The drawing under review shows one solid part. Ordinate dimensions are in mm from its lowest x, y, z. Round coordinates to 2 decimals unless told otherwise and drop trailing zeros. Order: outer loops, then holes, each group sorted by start corner. A loop starts at its lowest first (then second) coordinate and runs counter-clockwise, first axis right, second up. Notation, with made-up numbers: M 81.5,55 L 107.5,55 A27 ccw 107.5,92 Z; hole C -25,-18 d10. An arc over 180 degrees is marked long. Answer as a JSON object with one key per item and string values. Group by question number.
1) Consider section A-A, the plane x = 20. Write out the cut boundary in (y, z).
2) Consider section B-B, the plane z = 0.35. Write out the cut boundary in (x, y).
3) To check wall thickness, follow line 1 (Y direction, x = 60, z = 0.65); line 2 (X direction, y = 24, z = 0.8); line 3 (Y direction, x = 23, z = 0.35). State the ranges of each line that lie inside material, in increasing order.
4) Insertion check: pin 1 Ø7 at (x, y) = (60, 60) entering from -Z. The pin has a flat end and moves straight along its axis. Give the tip position at first contact, or say it passes through.
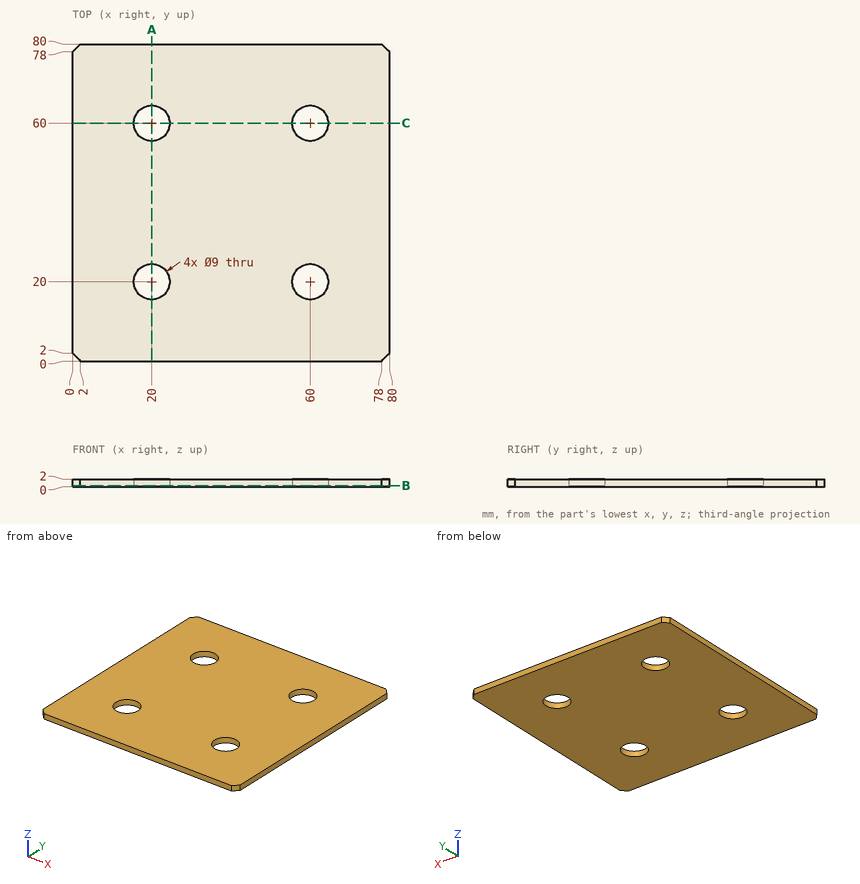
Results list:
{
 "1": {"outline": "M 0,0 L 15.5,0 L 15.5,2 L 0,2 Z; M 24.5,0 L 55.5,0 L 55.5,2 L 24.5,2 Z; M 64.5,0 L 80,0 L 80,2 L 64.5,2 Z"},
 "2": {"outline": "M 0,2 L 2,0 L 78,0 L 80,2 L 80,78 L 78,80 L 2,80 L 0,78 Z; hole C 20,20 d9; hole C 20,60 d9; hole C 60,20 d9; hole C 60,60 d9"},
 "3": {"line 1": "0 to 15.5, 24.5 to 55.5, 64.5 to 80", "line 2": "0 to 17.94, 22.06 to 57.94, 62.06 to 80", "line 3": "0 to 16.65, 23.35 to 56.65, 63.35 to 80"},
 "4": {"pin 1": "through"}
}
